Geometry: see drawing. Coordinates: mm, zero at the bounding-box minimum. A direction names the side the tool comes from. Round coordinates to 2 decimals unless told otherwise and drop trailing zeros. Loops run counter-clockwise (first coordinate to the right, second up) from the corner with the lowest first, then second, coordinate; pieces in that order, holes last.
(1) Cut plane D-D, the plane x = 6.5. Output: boundary loops of the cut face in (y, z).
(2) Access query for the marked faces 1, 2 and 3. Directions: +Z, -Z, +X, -X, +Y, -Y. A direction counts if a zero-diameter tool reaches every point of the face in a straight line with its end or side. Return the directions, or none.
(3) Cut plane A-A, the plane z = 4.7. Output: boundary loops of the cut face in (x, y).
(4) Line query: line 1 (X direction, y = 3.55, z = 4.7); line 2 (Z direction, x = 9.65, y = 2.65); line 3 (X direction, y = 3.4, z = 5.5). Output: solid intervals per line, ascending.
(5) Cut plane B-B, the plane y = 2.25. Output: boundary loops of the cut face in (x, z).
(6) Cut plane C-C, the plane x = 9. Output: boundary loops of the cut face in (y, z).
(7) First-contact query: pin 1 Ø0.6 at (x, z) = (11.5, 2.5) entering from -Y; pin 2 Ø0.6 at (x, z) = (4, 10.5) entering from -Y; pin 3 Ø1 at (x, y) = (9.5, 1) entering from +Z; pin 4 Ø1 at (x, z) = (9.5, 2) entering from +Y. Flat tips, straight axial feed; report the tip coordinate or a pass-through.
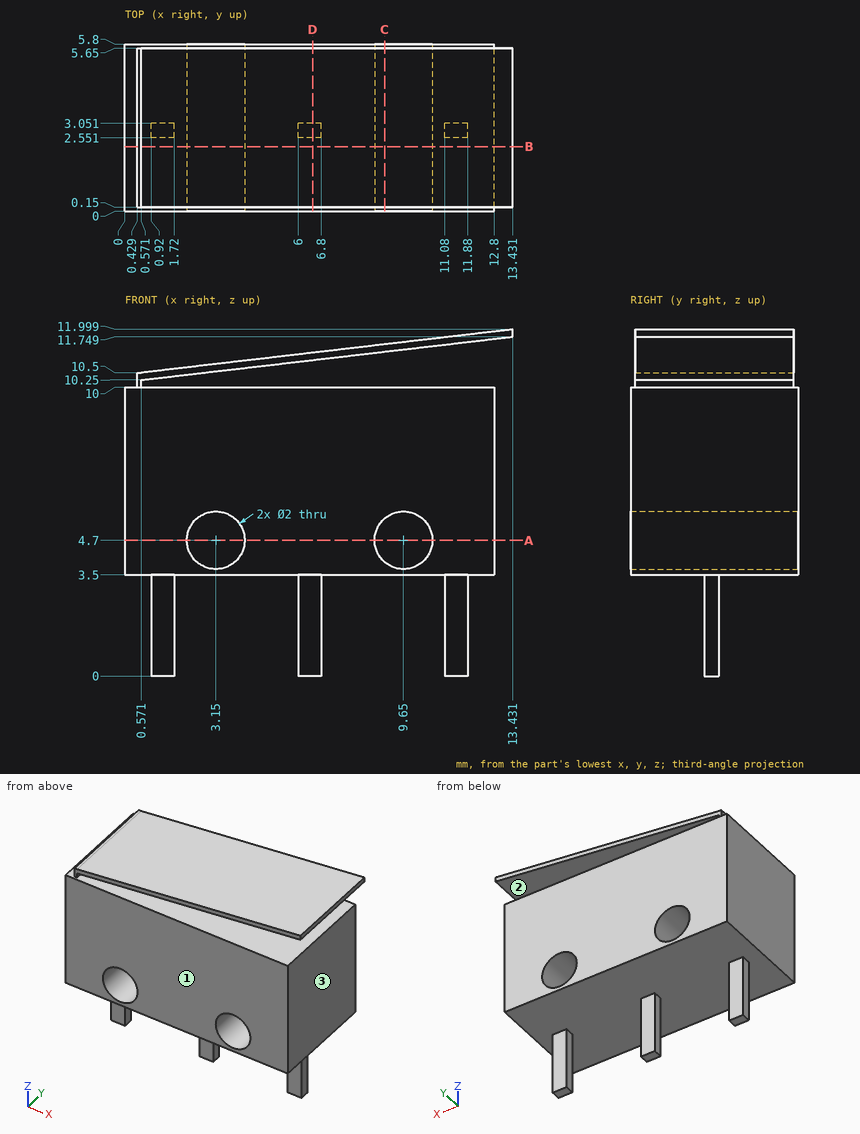
Reported:
1. outline: (0, 3.5) - (2.55, 3.5) - (2.55, 0) - (3.05, 0) - (3.05, 3.5) - (5.8, 3.5) - (5.8, 10) - (0, 10) - close; (0.15, 10.94) - (5.65, 10.94) - (5.65, 11.19) - (0.15, 11.19) - close
2. face 1: +Z, -Z, +X, -X, -Y
2. face 2: +X, +Y, -Y
2. face 3: -Z, +X, +Y, -Y
3. outline: (0, 0) - (2.15, 0) - (2.15, 5.8) - (0, 5.8) - close; (4.15, 0) - (8.65, 0) - (8.65, 5.8) - (4.15, 5.8) - close; (10.65, 0) - (12.8, 0) - (12.8, 5.8) - (10.65, 5.8) - close
4. line 1: x = 0 to 2.15, 4.15 to 8.65, 10.65 to 12.8
4. line 2: z = 3.5 to 3.7, 5.7 to 10, 11.31 to 11.56
4. line 3: x = 0 to 2.55, 3.75 to 9.05, 10.25 to 12.8
5. outline: (0, 3.5) - (12.8, 3.5) - (12.8, 10) - (0.57, 10) - (0.57, 10.25) - (13.43, 11.75) - (13.43, 12) - (0.57, 10.5) - (0.43, 10.5) - (0.43, 10) - (0, 10) - close; hole circle Ø2 at (3.15, 4.7); hole circle Ø2 at (9.65, 4.7)
6. outline: (0, 3.5) - (5.8, 3.5) - (5.8, 3.94) - (0, 3.94) - close; (0, 5.46) - (5.8, 5.46) - (5.8, 10) - (0, 10) - close; (0.15, 11.23) - (5.65, 11.23) - (5.65, 11.48) - (0.15, 11.48) - close
7. pin 1: stops at y = 2.55
7. pin 2: stops at y = 0.15
7. pin 3: stops at z = 11.6
7. pin 4: passes through
